```python
from build123d import *

# Parameters (mm, degrees)
SKETCH1_W                  = 381
SKETCH1_H                  = 177.8
PLATE_DEPTH                = 6.35
SKETCH4_R                  = 3.2639
CHASSISMOUNTINGHOLES_DEPTH = 6.35
SKETCH5_R                  = 2.5019
LEADSCREWGUIDEMOUNTS_DEPTH = 6.35
SKETCH6_R                  = 2.15265
LEADSCREWMOTORMOUNT_DEPTH  = 6.35


with BuildPart() as part:
    # Sketch1 → Plate (new body)
    with BuildSketch(Plane(origin=(0, 0, 0), x_dir=(1, 0, 0), z_dir=(0, 1, 0))):
        Rectangle(SKETCH1_W, SKETCH1_H)
    extrude(amount=PLATE_DEPTH)

    # Sketch4 → ChassisMountingHoles (cut)
    with BuildSketch(Plane.XZ):
        with Locations((0, 76.2)):
            Circle(SKETCH4_R)
        with Locations((-114.3, 76.2)):
            Circle(SKETCH4_R)
        with Locations((114.3, 76.2)):
            Circle(SKETCH4_R)
        with Locations((-114.3, -76.2)):
            Circle(SKETCH4_R)
        with Locations((114.3, -76.2)):
            Circle(SKETCH4_R)
    extrude(amount=-CHASSISMOUNTINGHOLES_DEPTH, mode=Mode.SUBTRACT)

    # Sketch5 → LeadScrewGuideMounts (cut)
    with BuildSketch(Plane.XZ):
        with Locations((171.45, 53.34)):
            Circle(SKETCH5_R)
        with Locations((171.45, 22.86)):
            Circle(SKETCH5_R)
        with Locations((-107.95, 53.34)):
            Circle(SKETCH5_R)
        with Locations((-107.95, 22.86)):
            Circle(SKETCH5_R)
        with Locations((171.45, -53.34)):
            Circle(SKETCH5_R)
        with Locations((171.45, -22.86)):
            Circle(SKETCH5_R)
        with Locations((-107.95, -22.86)):
            Circle(SKETCH5_R)
        with Locations((-107.95, -53.34)):
            Circle(SKETCH5_R)
    extrude(amount=-LEADSCREWGUIDEMOUNTS_DEPTH, mode=Mode.SUBTRACT)

    # Sketch6 → LeadScrewMotorMount (cut)
    with BuildSketch(Plane.XZ):
        with Locations((-171.45, 60.325)):
            Circle(SKETCH6_R)
        with Locations((-158.75, 60.325)):
            Circle(SKETCH6_R)
        with Locations((-171.45, 15.875)):
            Circle(SKETCH6_R)
        with Locations((-158.75, 15.875)):
            Circle(SKETCH6_R)
    extrude(amount=-LEADSCREWMOTORMOUNT_DEPTH, mode=Mode.SUBTRACT)


solid = part.part
```
Geometry check sheet. Reference: the model listing, model coordinates, mm. Round coordinates to 2 decimals unless told otherwise and drop trailing zeros. Use a Markdown table: item, result. Add a question column.
1) Thickness scan on line 1 along Z through (x, y) = (-107.95, 2.5); line 2 along Z through (x, y) = (-171.45, 2.5); line 3 along Z through (x, y) = (114.3, 3.75). Record the ranges inside material, lowest first.
2) Mould release check, pull along X, two halves, no side actions. Record for faces 1 (the cylindrical face through (-114.725, 3.131, -72.964)), 2 (the flat face through (-190.5, 3, 1)), 3 (the cylindrical face through (116.055, 3.131, -73.448)), 4 (the flat face through (-3, 6.35, -1)): released by +X, released by -X, zero draft, split by the parting line, or undercut.
3) Gauge pin test, flat end, axial feed: P1, Ø3, axis at x = 171.45, z = 22.86, coming from the -Y side. Record the tip position at first contact, or that the pin passes through.
Established:
| question | item | result |
|---|---|---|
| 1 | line 1 | -88.9 to -55.84, -50.84 to -25.36, -20.36 to 20.36, 25.36 to 50.84, 55.84 to 88.9 |
| 1 | line 2 | -88.9 to 13.72, 18.03 to 58.17, 62.48 to 88.9 |
| 1 | line 3 | -88.9 to -79.46, -72.94 to 72.94, 79.46 to 88.9 |
| 2 | face 1 | undercut |
| 2 | face 2 | released by -X |
| 2 | face 3 | undercut |
| 2 | face 4 | zero draft |
| 3 | P1 | through |
